Check sheet for the modelled part. Datum: model origin and axes. Units: mm. A direction names the side the tool comes from. Round coordinates to 2 decimals unless told otherwise and drop trailing zeros. Write each loop counter-clockwise with the first axis right and the second up, starting at its lowest first coordinate (ties: lowest second). Pieces come first, ordered by that corner, then holes. Notation, with made-up numbers: (-22.75, 13) -> (30.25, 13) arc R19 ccw to (30.25, 35) -> close; hole circle Ø9 at (83.5, 51.5). An arc over 180 degrees is marked (long way). Put each result on its own line as item: value. Start each with the question number.
from build123d import *

# Parameters (mm, degrees)
SKETCH_1_R             = 19.325
SKETCH_1_R_2           = 2.5
EXTRUDE_1_DEPTH        = 16
SKETCH_2_R             = 22.5
SKETCH_2_R_2           = 2.5
EXTRUDE_2_DEPTH        = 2
SKETCH_3_R             = 22.5
SKETCH_3_R_2           = 2.5
EXTRUDE_3_DEPTH        = 2
SKETCH_4_R             = 5.5
CUT_EXTRUDE_1_DEPTH    = 20
HOLE_WIZARD_M3_1_D     = 2.5
HOLE_WIZARD_M3_1_DEPTH = 8.5
HOLE_WIZARD_M3_1_TIP   = 0.751075774
SKETCH_7_R             = 9.5
CUT_EXTRUDE_3_DEPTH    = 5
SKETCH_8_R             = 8
CUT_EXTRUDE_4_DEPTH    = 2.5


with BuildPart() as part:
    # 草图1 → 凸台-拉伸1 (new body)
    with BuildSketch(Plane(origin=(0, 0, 0), x_dir=(1, 0, 0), z_dir=(0, 1, 0))):
        Circle(SKETCH_1_R)
        Circle(SKETCH_1_R_2, mode=Mode.SUBTRACT)
    extrude(amount=EXTRUDE_1_DEPTH)

    # 草图2 → 凸台-拉伸2 (add)
    with BuildSketch(Plane(origin=(0, 16, 0), x_dir=(1, 0, 0), z_dir=(0, 1, 0))):
        Circle(SKETCH_2_R)
        Circle(SKETCH_2_R_2, mode=Mode.SUBTRACT)
    extrude(amount=EXTRUDE_2_DEPTH)

    # 草图3 → 凸台-拉伸3 (add)
    with BuildSketch(Plane.XZ):
        Circle(SKETCH_3_R)
        Circle(SKETCH_3_R_2, mode=Mode.SUBTRACT)
    extrude(amount=EXTRUDE_3_DEPTH)

    # 草图4 → 切除-拉伸1 (cut)
    with BuildSketch(Plane.XZ.offset(2)):
        Circle(SKETCH_4_R)
    extrude(amount=-CUT_EXTRUDE_1_DEPTH, mode=Mode.SUBTRACT)

    # M3 螺纹孔1
    with Locations(Plane(origin=(0, -2, 8), x_dir=(0, 0, -1), z_dir=(0, -1, 0))):
        with Locations((0, 0), (8, 8), (16, 0), (8, -8)):
            Hole(HOLE_WIZARD_M3_1_D / 2, depth=HOLE_WIZARD_M3_1_DEPTH)
            with Locations((0, 0, -(HOLE_WIZARD_M3_1_DEPTH + HOLE_WIZARD_M3_1_TIP / 2))):  # 118° drill point
                Cone(0, HOLE_WIZARD_M3_1_D / 2, HOLE_WIZARD_M3_1_TIP, mode=Mode.SUBTRACT)

    # 草图7 → 切除-拉伸3 (cut)
    with BuildSketch(Plane(origin=(0, 18, 0), x_dir=(1, 0, 0), z_dir=(0, 1, 0))):
        Circle(SKETCH_7_R)
    extrude(amount=-CUT_EXTRUDE_3_DEPTH, mode=Mode.SUBTRACT)

    # 草图8 → 切除-拉伸4 (cut)
    with BuildSketch(Plane(origin=(0, 13, 0), x_dir=(1, 0, 0), z_dir=(0, 1, 0))):
        Circle(SKETCH_8_R)
    extrude(amount=-CUT_EXTRUDE_4_DEPTH, mode=Mode.SUBTRACT)


solid = part.part
1. Material ranges on L1, parallel to Z at x = 0, y = 1.25 (3 decimals); L2, parallel to X at y = 14.2, z = 0 (3 decimals); L3, parallel to Z at x = 0, y = 11.7 (3 decimals), recorded low to high. Write a range as [from, to].
2. Section check D-D, the plane x = 10.5. Enter the section's corners in (y, z).
3. Access from +Z, -Z, +X, -X, +Y, -Y to the whole of each face (thin tool, end or side, straight path). Record for faces 5 (the cylindrical face through (-1.73, 11.77, 7.81)), 6 (the cylindrical face through (6.78, 2.31, -0.27)), 7 (the flat face through (10, 16, -17)).
4. Draft check along X on faces 1 (the cylindrical face through (-9.22, 2.31, -0.27)), 2 (the cylindrical face through (-19.306, 7.888, -0.85)), 3 (the flat face through (-4.3, 13, 7)), 4 (the flat face through (10, 0, 17)). Enter one of: released by +X, released by -X, zero draft, split by the parting line, or undercut.
5. Section check C-C, the plane x = 18.5. Enter the section's corners in (y, z).
6. Gauge pin test, flat ends, axial feed: P1, Ø1.5, axis at y = 14, z = 12.5, coming from the +X side; P2, Ø4, axis at x = 0, z = 8, coming from the -Y side; P3, Ø5, axis at x = -2, z = 3.5, coming from the +Y side; P4, Ø1.5, axis at x = -8, z = 0, coming from the -Y side. Record the tip position at first contact, or that the pin passes through.
7. Section check A-A, the plane y = 4.75. Enter the section's corners in (x, z) (3 decimals), then the cut area to 3 significant figures.
8. Section check B-B, the plane y = 9.5. Enter the section's corners in (x, z) (3 decimals), then the cut area to 3 significant figures.
Reply:
1. L1: z = [-19.325, -9.25], [-6.75, -5.5], [5.5, 6.75], [9.25, 19.325]
1. L2: x = [-19.325, -9.5], [9.5, 19.325]
1. L3: z = [-19.325, -8], [8, 19.325]
2. outline: (-2, -19.9) -> (0, -19.9) -> (0, -16.22) -> (16, -16.22) -> (16, -19.9) -> (18, -19.9) -> (18, 19.9) -> (16, 19.9) -> (16, 16.22) -> (0, 16.22) -> (0, 19.9) -> (-2, 19.9) -> close
3. face 5: +Y
3. face 6: -Y
3. face 7: none
4. face 1: undercut
4. face 2: split by the parting line
4. face 3: undercut
4. face 4: zero draft
5. outline: (-2, -12.81) -> (0, -12.81) -> (0, -5.59) -> (16, -5.59) -> (16, -12.81) -> (18, -12.81) -> (18, 12.81) -> (16, 12.81) -> (16, 5.59) -> (0, 5.59) -> (0, 12.81) -> (-2, 12.81) -> close
6. P1: stops at x = 15.34
6. P2: stops at y = -2
6. P3: stops at y = 10.5
6. P4: stops at y = 6.8
7. outline: circle Ø38.65 at (0, 0); hole circle Ø2.5 at (-8, 0); hole circle Ø11 at (0, 0); hole circle Ø2.5 at (0, -8); hole circle Ø2.5 at (0, 8); hole circle Ø2.5 at (8, 0)
7. area: 1,060 mm2
8. outline: circle Ø38.65 at (0, 0); hole circle Ø11 at (0, 0)
8. area: 1,080 mm2
